For this review, take the finished solid that the model builds, in its own axes (mm). A direction names the side the tool comes from. Coordinates: 2 decimals unless noted, no trailing zeros. Write each loop counter-clockwise with the first axis right and the second up, starting at its lowest first coordinate (ties: lowest second). Pieces come first, ordered by that corner, then holes.
1) We need section D-D on z = 23.5. Write out the cut boundary in (x, y) (3 decimals), then the cut area to 3 significant figures.
2) Mouldability with a two-part tool opening along X and no side actions: class faces 1 (the face through (-57.15, -1, 16)), 2 (the face through (-0.8, 53.975, 1.5)), 3 (the face through (-13, -52.225, 7)) as pulls with the +X half, pulls with the -X half, needs draft (parallel to the pull), parting line crosses it, or undercut.
3) We need section B-B on z = 10. Write out the cut boundary in (x, y) (3 decimals), then the cut area to 3 significant figures.
4) To check wall thickness, follow line 1 along X through (y, z) = (-17, 17); line 2 along Y through (x, z) = (-27, 20) (3 decimals); line 3 along Z through (x, y) = (-26.5, 34.5). State the ranges of each line that lie inside material, in increasing order.
5) Insertion check: P1, Ø15, axis at x = 7.5, z = 17.5, coming from the +Y side; P2, Ø4, axis at x = -36.5, y = -8.5, coming from the +Z side. Each pin has a flat end and moves straight along its axis. Give the tip position at first contact, or say it passes through.
6) We need section A-A on x = 0. Write out the cut boundary in (y, z) (3 decimals), then the cut area to 3 significant figures.
7) We need section C-C on y = 20. Write out the cut boundary in (x, z), then the cut area to 3 significant figures.
8) For faces 4 (the face through (-1, 1, 1.75)), 5 (the face through (-0.8, -53.975, 1.5)), list the 3-axis set-ups (+Z, -Z, +X, -X, +Y, -Y) from which the entire face can be reached by the end or side of a thin tool; tool diameter is ignored.
from build123d import *

# Parameters (mm, degrees)
F0_W     = 114.3
F0_H     = 107.95
F1_DEPTH = 31.75
F3_T     = -1.75
F4_DEPTH = 1.75


# Not quite as in the source:
# - a pattern or mirror of a feature is missing from the dataset's text; its kind, count and spacing are read off the source's solid


with BuildPart() as f1:
    # F0 (on Top) → F1 (new body)
    with BuildSketch(Plane.XY):
        Rectangle(F0_W, F0_H)
    extrude(amount=F1_DEPTH)

    # F3
    f3_openings = [f1.faces().sort_by_distance(p)[0] for p in [
        (0, 0, 31.75),
    ]]
    offset(amount=F3_T, openings=f3_openings)

    # F2 (on face) → F4 (cut)
    with BuildSketch(Plane.XZ.offset(53.975)):
        with BuildLine():
            ThreePointArc((-7.7136243103, 31.75), (-13.7391570489, 25.8280615857), (-15.873456613, 17.6536402154))
            ThreePointArc((-15.873456613, 17.6536402154), (0, 2), (15.873456613, 17.6536402154))
            Line((15.873456613, 17.6536402154), (15.873456613, 18.0963597846))
            ThreePointArc((15.873456613, 18.0963597846), (13.6269244294, 26.0188661333), (7.7136243103, 31.75))
            Line((7.7136243103, 31.75), (-7.7136243103, 31.75))
        make_face()
        with BuildLine():
            Line((-16.0700342862, 31.75), (-15.873456613, 17.6536402154))
            ThreePointArc((-15.873456613, 17.6536402154), (-13.7391570489, 25.8280615857), (-7.7136243103, 31.75))
            Line((-7.7136243103, 31.75), (-16.0700342862, 31.75))
        make_face()
        with BuildLine():
            Line((15.873456613, 18.0963597846), (15.873456613, 17.6536402154))
            ThreePointArc((15.873456613, 17.6536402154), (15.8746141486, 17.7643174175), (15.875, 17.875))
            ThreePointArc((15.875, 17.875), (15.8746141486, 17.9856825825), (15.873456613, 18.0963597846))
        make_face()
        with BuildLine():
            ThreePointArc((7.7136243103, 31.75), (0, 33.75), (-7.7136243103, 31.75))
            Line((-7.7136243103, 31.75), (7.7136243103, 31.75))
        make_face()
        with BuildLine():
            ThreePointArc((7.7136243103, 31.75), (13.6269244294, 26.0188661333), (15.873456613, 18.0963597846))
            Line((15.873456613, 18.0963597846), (15.873456613, 31.75))
            Line((15.873456613, 31.75), (7.7136243103, 31.75))
        make_face()
    f4 = extrude(amount=-F4_DEPTH, mode=Mode.SUBTRACT)

    # F4_copies: F4 across plane
    add(f4.mirror(Plane.ZX), mode=Mode.SUBTRACT)


solid = f1.part
Result:
1. outline: (-57.15, -53.975) - (-15.955, -53.975) - (-15.955, -52.225) - (-55.4, -52.225) - (-55.4, 52.225) - (-15.955, 52.225) - (-15.955, 53.975) - (-57.15, 53.975) - close; (15.873, -53.975) - (57.15, -53.975) - (57.15, 53.975) - (15.873, 53.975) - (15.873, 52.225) - (55.4, 52.225) - (55.4, -52.225) - (15.873, -52.225) - close
1. area: 654 mm2
2. face 1: pulls with the -X half
2. face 2: needs draft
2. face 3: undercut
3. outline: (-57.15, -53.975) - (-13.784, -53.975) - (-13.784, -52.225) - (-55.4, -52.225) - (-55.4, 52.225) - (-13.784, 52.225) - (-13.784, 53.975) - (-57.15, 53.975) - close; (13.784, -53.975) - (57.15, -53.975) - (57.15, 53.975) - (13.784, 53.975) - (13.784, 52.225) - (55.4, 52.225) - (55.4, -52.225) - (13.784, -52.225) - close
3. area: 669 mm2
4. line 1: x = -57.15 to -55.4, 55.4 to 57.15
4. line 2: y = -53.975 to -52.225, 52.225 to 53.975
4. line 3: z = 0 to 1.75
5. P1: passes through
5. P2: stops at z = 1.75
6. outline: (-53.975, 0) - (53.975, 0) - (53.975, 2) - (52.225, 2) - (52.225, 1.75) - (-52.225, 1.75) - (-52.225, 2) - (-53.975, 2) - close
6. area: 190 mm2
7. outline: (-57.15, 0) - (57.15, 0) - (57.15, 31.75) - (55.4, 31.75) - (55.4, 1.75) - (-55.4, 1.75) - (-55.4, 31.75) - (-57.15, 31.75) - close
7. area: 305 mm2
8. face 4: +Z
8. face 5: +Z, -Z, +X, -X, -Y
